Verification items for this drawing (mm, ordinates from the low corner). Give positions to 0.01 mm unless a question says otherwise; leave off trailing zeros. Order: outer loops, then holes, each group sorted by start corner. A loop starts at its lowest first (then second) coordinate and runs counter-clockwise, first axis right, second up. Notation, with made-up numbers: M -10.75,64.5 L 13.25,64.5 A11 ccw 13.25,70.5 Z; hole C 79.5,87.25 d10. An arc over 180 degrees is marked long. Answer as a JSON object with one key per item and string values.
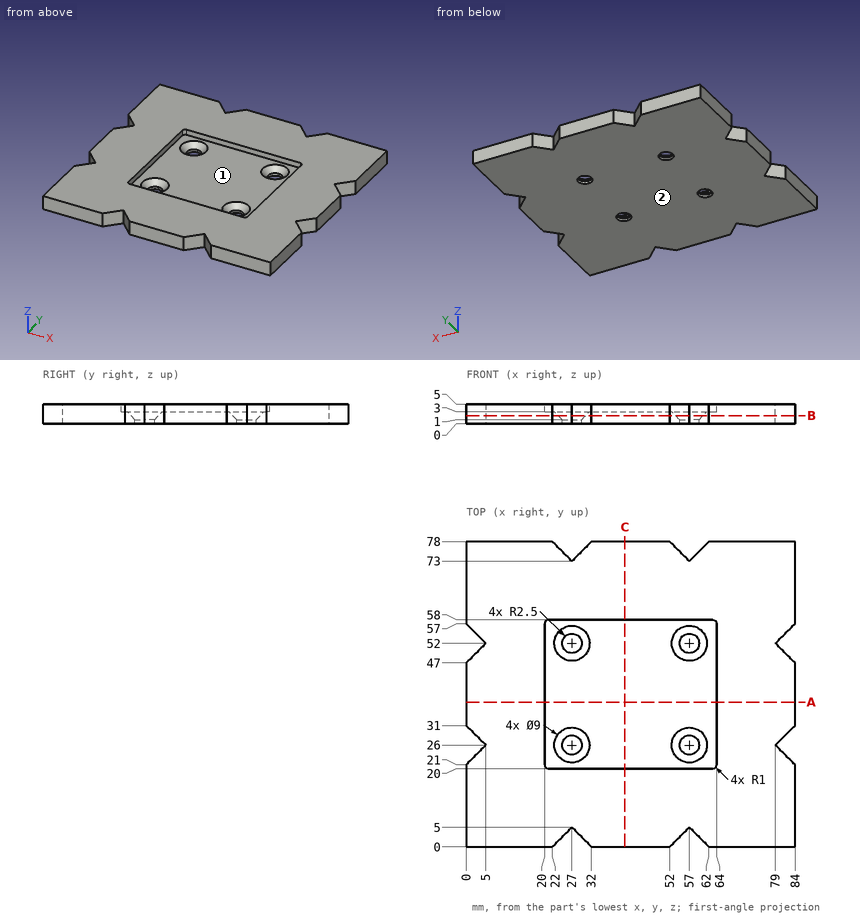
Q1. Section check A-A on y = 37. Record the cut outline in (x, z), then the cut area to 3 significant figures.
Resolved:
{"outline": "M 0,0 L 84,0 L 84,5 L 64,5 L 64,3 L 20,3 L 20,5 L 0,5 Z", "area": "332 mm²"}
Q2. Section check C-C on x = 40.5. Record the cut outline in (y, z), then the cut area to 3 significant figures.
Resolved:
{"outline": "M 0,0 L 78,0 L 78,5 L 58,5 L 58,3 L 20,3 L 20,5 L 0,5 Z", "area": "314 mm²"}
Q3. Gauge pin test, flat end, axial feed: pin 1 Ø19 at (x, y) = (37, 41) entering from +Z. Record the tip position at first contact, or that the pin passes through.
Resolved:
{"pin 1": "stops at z = 3"}
Q4. Release check for a two-part mould opening along Y. For the marked faces 1 and 2 record: +Y half, -Y half, draft (parallel to the pull), parting line (faces both ways), or undercut.
Resolved:
{"face 1": "undercut", "face 2": "draft"}
Q5. Material ranges on L1, parallel to X at y = 44, z = 3.3; L2, parallel to Y at x = 79.5, z = 2.2; L3, parallel to X at y = 26.5, z = 2.9, recorded low to high.
Resolved:
{"L1": "x = 0 to 20, 64 to 84", "L2": "y = 0 to 25.5, 26.5 to 51.5, 52.5 to 78", "L3": "x = 4.5 to 22.63, 31.37 to 52.63, 61.37 to 79.5"}
Q6. Section check B-B on z = 2. Count the separate pieces of the cut face and the enclosed holes in it, then the cut area to 3 significant figures.
Resolved:
{"separate pieces": "1", "enclosed holes": "4", "area": "6,200 mm²"}
